Geometry check sheet. Reference: drawing and pictorial views, mm from the part's lowest x, y, z. A direction names the side the tool comes from. Give positions to 0.01 mm unless a question says otherwise; leave off trailing zeros. Write each loop counter-clockwise with the first axis right and the second up, starting at its lowest first coordinate (ties: lowest second). Pieces come first, ordered by that corner, then holes. Notation, with made-up numbers: (-31.5, 76) - (-22.5, 76) arc R29 ccw to (-22.5, 101) - close; hole circle Ø1 at (2, 77). An arc over 180 degrees is marked (long way). Put each result on its own line as item: value.
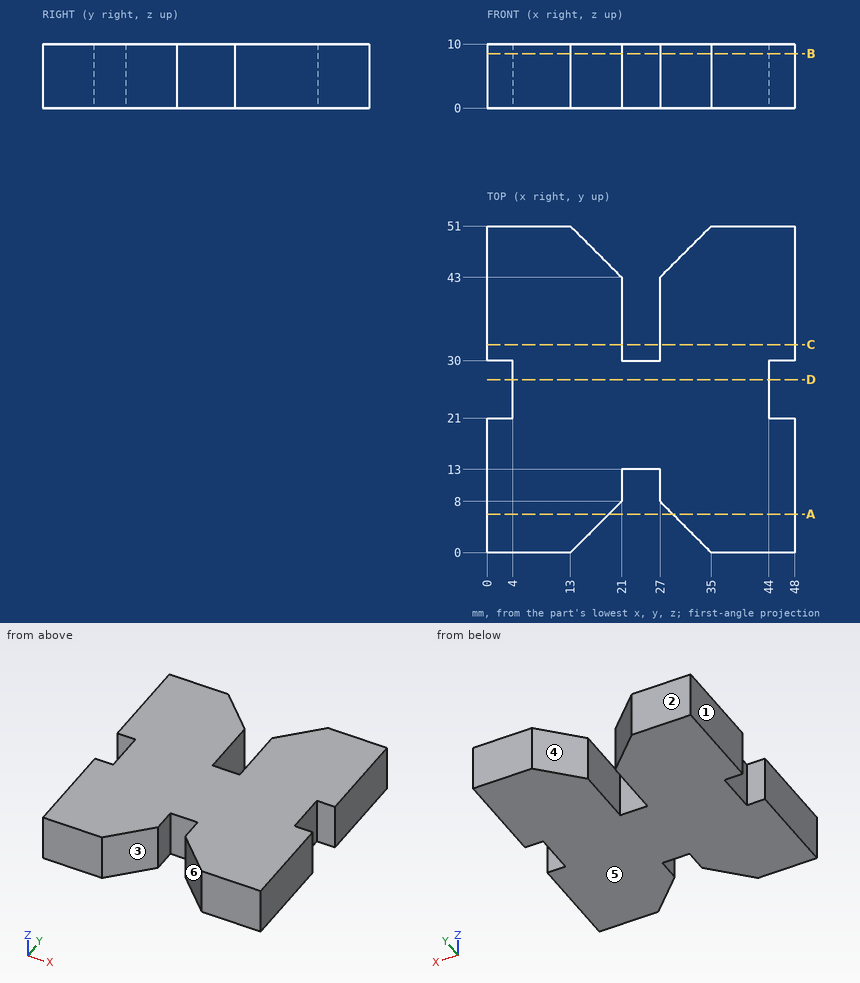
Q1. Go/stop test with flat-tipped pins: pin 1 Ø4 at (x, y) = (24.5, 30) entering from -Z; pin 2 Ø1.8 at (x, z) = (24.5, 4) entering from -Y. Record where each tip stops, or that it passes through.
Answers follow:
pin 1: stops at z = 0
pin 2: stops at y = 13
Q2. Set-up check for the marked faces 4, 5 and 6: record each of +Z, -Z, +X, -X, +Y, -Y from which the full face is reachable in a straight line by a thin tool's end or side.
Answers follow:
face 4: +Z, -Z, +Y
face 5: -Z, +X, -X, +Y, -Y
face 6: +Z, -Z, -Y
Q3. Section check C-C, the plane y = 32.5. Record the cut outline in (x, z), plus the area to 3 significant figures.
Answers follow:
outline: (0, 0) - (21, 0) - (21, 10) - (0, 10) - close; (27, 0) - (48, 0) - (48, 10) - (27, 10) - close
area: 420 mm2
Q4. Section check A-A, the plane y = 6. Record the cut outline in (x, z), plus the area to 3 significant figures.
Answers follow:
outline: (0, 0) - (19, 0) - (19, 10) - (0, 10) - close; (29, 0) - (48, 0) - (48, 10) - (29, 10) - close
area: 380 mm2
Q5. Section check B-B, the plane z = 8.5. Record the cut outline in (x, y).
Answers follow:
outline: (0, 0) - (13, 0) - (21, 8) - (21, 13) - (27, 13) - (27, 8) - (35, 0) - (48, 0) - (48, 21) - (44, 21) - (44, 30) - (48, 30) - (48, 51) - (35, 51) - (27, 43) - (27, 30) - (21, 30) - (21, 43) - (13, 51) - (0, 51) - (0, 30) - (4, 30) - (4, 21) - (0, 21) - close
Q6. Release check for a two-part mould opening along X. For the marked faces 1, 2 and 3 record: released by +X, released by -X, zero draft, split by the parting line, or undercut.
Answers follow:
face 1: released by -X
face 2: zero draft
face 3: undercut
Q7. Section check D-D, the plane y = 27. Record the cut outline in (x, z), plus the area to 3 significant figures.
Answers follow:
outline: (4, 0) - (44, 0) - (44, 10) - (4, 10) - close
area: 400 mm2
Q8. Scan lines: line 1 along X through (y, z) = (42.5, 1.5); line 2 along Y through (x, z) = (46, 6.5); line 3 along X through (y, z) = (21.5, 7). Record each from-to range of solid material in increasing order.
Answers follow:
line 1: x = 0 to 21, 27 to 48
line 2: y = 0 to 21, 30 to 51
line 3: x = 4 to 44
